Geometry: final body of the model. Coordinates: model frame, mm. Face numbers are marked on the shaded views. A direction names the side the tool comes from. Round coordinates to 2 decimals unless told otherwise and drop trailing zeros. Loops run counter-clockwise (first coordinate to the right, second up) from the corner with the lowest first, then second, coordinate; pieces in that order, holes last. Notation, with made-up numbers: M -21.75,35.5 L 17.25,35.5 A33 cw 17.25,70.5 Z; hole C -34.5,44.25 d10. An arc over 180 degrees is marked long. Return JSON: item names as keys, results as strings.
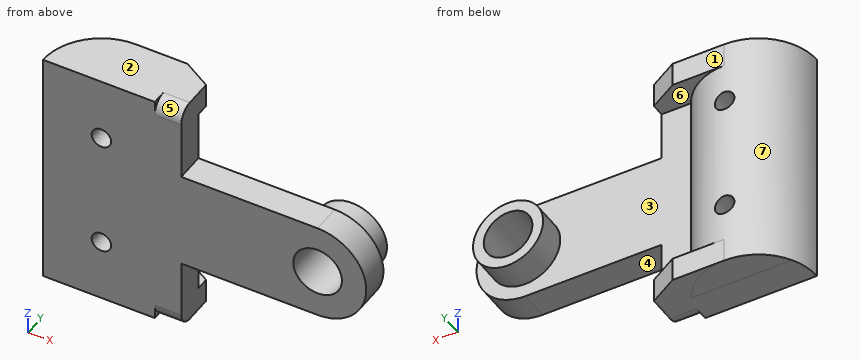
from build123d import *

# Parameters (mm, degrees)
CROQUIS1_R              = 2.500000266
CROQUIS1_R_2            = 1.000000047
CROQUIS1_R_3            = 1.000000141
SALIENTE_EXTRUIR1_DEPTH = 3
SALIENTE_EXTRUIR2_DEPTH = 24.95
CROQUIS3_W              = 8.200000763
CROQUIS3_H              = 2.45
SALIENTE_EXTRUIR3_DEPTH = 3
CORTAR_EXTRUIR1_DEPTH   = 31
CORTAR_EXTRUIR2_DEPTH   = 2.72
CROQUIS6_R              = 3.6
CROQUIS6_R_2            = 2.500000266
SALIENTE_EXTRUIR4_DEPTH = 3
CORTAR_EXTRUIR3_DEPTH   = 27
CROQUIS8_R              = 1.000000047
CROQUIS8_R_2            = 1.000000141
CORTAR_EXTRUIR4_DEPTH   = 27


with BuildPart() as part:
    # Croquis1 → Saliente-Extruir1 (new body)
    with BuildSketch(Plane(origin=(0, 0, 0), x_dir=(1, 0, 0), z_dir=(0, 1, 0))):
        with BuildLine():
            Line((-16.847731683, 12.84659639), (-2.64773092, 12.84659639))
            Line((-2.64773092, 12.84659639), (-2.64773092, 5.396596581))
            Line((-2.64773092, 5.396596581), (11.352269703, 5.396596581))
            ThreePointArc((11.352269703, 5.396596581), (16.352269703, 0.396596581), (11.352269703, -4.603403419))
            Line((11.352269703, -4.603403419), (-2.64773092, -4.603403419))
            Line((-2.64773092, -4.603403419), (-2.64773092, -12.103403419))
            Line((-2.64773092, -12.103403419), (-16.847731683, -12.103403419))
            Line((-16.847731683, -12.103403419), (-16.847731683, 12.84659639))
        make_face()
        with Locations((11.352269089, 0.39659652)):
            Circle(CROQUIS1_R, mode=Mode.SUBTRACT)
        with Locations((-10.847731494, 6.396596534)):
            Circle(CROQUIS1_R_2, mode=Mode.SUBTRACT)
        with Locations((-10.847730816, -5.603403561)):
            Circle(CROQUIS1_R_3, mode=Mode.SUBTRACT)
    extrude(amount=SALIENTE_EXTRUIR1_DEPTH)

    # Croquis2 → Saliente-Extruir2 (add)
    with BuildSketch(Plane.XY.offset(12.103403419)):
        with BuildLine():
            Line((-16.043884106, 3), (-5.651579261, 3))
            ThreePointArc((-5.651579261, 3), (-10.847731683, 6), (-16.043884106, 3))
        make_face()
    extrude(amount=-SALIENTE_EXTRUIR2_DEPTH)

    # Croquis3 → Saliente-Extruir3 (add)
    with BuildSketch(Plane(origin=(0, 3, 0), x_dir=(1, 0, 0), z_dir=(0, 1, 0))):
        with Locations((-6.747731302, 11.62159639)):
            Rectangle(CROQUIS3_W, CROQUIS3_H)
        with Locations((-6.747731302, -10.878403419)):
            Rectangle(CROQUIS3_W, CROQUIS3_H)
    extrude(amount=SALIENTE_EXTRUIR3_DEPTH)

    # Croquis4 → Cortar-Extruir1 (cut)
    with BuildSketch(Plane.XY.offset(12.103403419)):
        Polygon((-2.64773092, 4.33), (-2.64773092, 6), (-5.53773092, 6), align=None)
    extrude(amount=-CORTAR_EXTRUIR1_DEPTH, mode=Mode.SUBTRACT)

    # Croquis5 → Cortar-Extruir2 (cut)
    with BuildSketch(Plane(origin=(-2.64773092, 0, 0), x_dir=(0, 0, -1), z_dir=(1, 0, 0))):
        with BuildLine():
            Line((12.84659639, 1.5), (14.964292121, 1.5))
            ThreePointArc((14.964292121, 1.5), (0, -14.850313202), (-14.964292121, 1.5))
            Line((-14.964292121, 1.5), (-12.103403419, 1.5))
            ThreePointArc((-12.103403419, 1.5), (-11.664063591, 0.439339828), (-10.603403419, 0))
            Line((-10.603403419, 0), (11.34659639, 0))
            ThreePointArc((11.34659639, 0), (12.407256562, 0.439339828), (12.84659639, 1.5))
        make_face()
    extrude(amount=-CORTAR_EXTRUIR2_DEPTH, mode=Mode.SUBTRACT)

    # Croquis6 → Saliente-Extruir4 (add)
    with BuildSketch(Plane(origin=(0, 3, 0), x_dir=(1, 0, 0), z_dir=(0, 1, 0))):
        with Locations((11.352269089, 0.39659652)):
            Circle(CROQUIS6_R)
        with Locations((11.352269089, 0.39659652)):
            Circle(CROQUIS6_R_2, mode=Mode.SUBTRACT)
    extrude(amount=SALIENTE_EXTRUIR4_DEPTH)

    # Croquis7 → Cortar-Extruir3 (cut)
    with BuildSketch(Plane.XY.offset(12.103403419)):
        with BuildLine():
            Line((-12.758872324, 7.288729336), (-12.369518171, 5.803806155))
            ThreePointArc((-12.369518171, 5.803806155), (-15.59803267, 3.665329526), (-16.847731683, 0))
            Line((-16.847731683, 0), (-18.382851714, 0))
            ThreePointArc((-18.382851714, 0), (-16.813413036, 4.603116322), (-12.758872324, 7.288729336))
        make_face()
    extrude(amount=-CORTAR_EXTRUIR3_DEPTH, mode=Mode.SUBTRACT)

    # Croquis8 → Cortar-Extruir4 (cut)
    with BuildSketch(Plane.XZ):
        with Locations((-10.847731494, -6.396596534)):
            Circle(CROQUIS8_R)
        with Locations((-10.847730816, 5.603403561)):
            Circle(CROQUIS8_R_2)
    extrude(amount=-CORTAR_EXTRUIR4_DEPTH, mode=Mode.SUBTRACT)


solid = part.part
Q1. Section query C-C (z = 5). Output: boundary loops of the cut face in (x, y), plus the area to 3 significant figures.
Determined:
{"outline": "M -16.85,0 L -11.65,0 L -11.65,5.95 A6 ccw Z; M -10.05,0 L -2.65,0 L -2.65,3 L -5.65,3 A6 ccw -10.05,5.95 Z", "area": "54.4 mm^2"}
Q2. Pin query (flat end, axial travel): pin 1 (0.9 mm diameter, centred on x = 7, y = 1.5, fed in from +Z); pin 2 (2 mm diameter, centred on y = 2.5, z = -8, fed in from +X); pin 3 (2.5 mm diameter, centred on x = 4, y = 1.5, fed in from -Z). Return the tip coordinate at first contact, or that it passes through.
Determined:
{"pin 1": "stops at z = 4.6", "pin 2": "stops at x = -2.65", "pin 3": "stops at z = -5.4"}
Q3. Section query B-B (x = 12). Output: boundary loops of the cut face in (y, z).
Determined:
{"outline": "M 0,-5.35 L 3,-5.35 L 3,-3.94 L 6,-3.94 L 6,-2.81 L 0,-2.81 Z; M 0,2.02 L 6,2.02 L 6,3.14 L 3,3.14 L 3,4.56 L 0,4.56 Z"}
Q4. Pull-direction query (Z, two-part tool) for the marked faces 1, 2 and 3; classes: pulls with the +Z half, pulls with the -Z half, needs draft (parallel to the pull), parting line crosses it, or undercut.
Determined:
{"face 1": "needs draft", "face 2": "pulls with the +Z half", "face 3": "undercut"}
Q5. Section query D-D (z = 1.75). Output: boundary loops of the cut face in (x, y).
Determined:
{"outline": "M -16.85,0 L 10.07,0 L 10.07,6 L 8.46,6 L 8.46,3 L -5.65,3 A6 ccw Z; M 12.63,0 L 15.87,0 L 15.87,3 L 14.24,3 L 14.24,6 L 12.63,6 Z"}
Q6. Section query A-A (y = 3.5). Output: boundary loops of the cut face in (x, z).
Determined:
{"outline": "M -15.72,-12.85 L -2.65,-12.85 L -2.65,-10.4 L -5.97,-10.4 L -5.97,9.65 L -2.65,9.65 L -2.65,12.1 L -15.72,12.1 Z; C 11.35,-0.4 d7.2; hole C -10.85,-6.4 d2; hole C -10.85,5.6 d2; hole C 11.35,-0.4 d5"}
Q7. Material intervals for L1, parallel to X at y = 3.25, z = -0.25; L2, parallel to Y at x = 13.5, z = -4.5; L3, parallel to Z at x = -6, y = 5.5, sorted ascending.
Determined:
{"L1": "x = -15.89 to -5.8, 7.76 to 8.86, 13.85 to 14.95", "L2": "y = 0 to 3", "L3": "z = -12.85 to -10.4, 9.65 to 12.1"}
Q8. Reachability of the marked faces 4, 5, 6 and 7 from +Z, -Z, +X, -X, +Y, -Y: full face, straight path, thin tool, end or side. Return the list, or none.
Determined:
{"face 4": "-Z, +X, +Y, -Y", "face 5": "+Z, +X, -Y", "face 6": "+X, +Y", "face 7": "+Y"}
